Work out the finished part from the listing and answer in its coordinate system (mm). A direction names the side the tool comes from. Round coordinates to 2 decimals unless told otherwise and drop trailing zeros. Order: outer loops, then holes, each group sorted by start corner. A loop starts at its lowest first (then second) coordinate and runs counter-clockwise, first axis right, second up. Notation, with made-up numbers: (72.25, 29) - (80.25, 29) arc R32 ccw to (80.25, 62) - close; hole circle Ø9 at (62, 86.25). An arc over 180 degrees is marked (long way). Use CSV: the item, a comma, the result in double quotes.
from build123d import *

# Parameters (mm, degrees)
F1_DEPTH = 35
F2_W     = 220
F2_H     = 315
F3_DEPTH = 5


with BuildPart() as f1:
    # F0 (on Front) → F1 (new body)
    with BuildSketch(Plane.XZ):
        Polygon((-110, -157.5), (110, -157.5), (110, 157.5), (-110, 157.5), (-110, 152.500004), (105.000004, 152.500004), (105.000004, -152.500004), (-110, -152.500004), align=None)
    extrude(amount=F1_DEPTH)

    # F2 (on face) → F3 (join)
    with BuildSketch(Plane.XZ.offset(35)):
        Rectangle(F2_W, F2_H)
    extrude(amount=F3_DEPTH)


solid = f1.part
(1) Find the intervals of material crossed by L1, parallel to Z at x = -84.5, y = -26; L2, parallel to Y at x = -98, z = -5; L3, parallel to X at y = -19, z = -26, in increasing order. Write a range as from..to.
Findings below:
L1,"z = -157.5..-152.5, 152.5..157.5"
L2,"y = -40..-35"
L3,"x = 105..110"
(2) The mould has two halves that part along Z. Classify faces 3 (the flat face through (-2, -20, 157.5)), 4 (the flat face through (-4, -17, 152.5)), 5 (the flat face through (-2, -40, 2)): released by +Z, released by -Z, zero draft, split by the parting line, or undercut.
Findings below:
face 3,"released by +Z"
face 4,"undercut"
face 5,"zero draft"
(3) For faces 1 (the flat face through (105.4, 0, 0.7)), 2 (the flat face through (-1, -17, -152.5)), determine the directions among +Z, -Z, +X, -X, +Y, -Y from which every point of the face is accessible in a straight line to the end or side of a thin tool.
Findings below:
face 1,"+Z, -Z, +X, -X, +Y"
face 2,"-X, +Y"
(4) Find section C-C (z = -17.5). Determine the outline of the cut face in (x, y).
Findings below:
outline,"(-110, -40) - (110, -40) - (110, 0) - (105, 0) - (105, -35) - (-110, -35) - close"
(5) Find section B-B (y = -22). Determine the outline of the cut face in (x, z), and give its area (4 significant figures).
Findings below:
outline,"(-110, -157.5) - (110, -157.5) - (110, 157.5) - (-110, 157.5) - (-110, 152.5) - (105, 152.5) - (105, -152.5) - (-110, -152.5) - close"
area,"3,725 mm²"
(6) Each of these flat-tipped pins is pushed along its axis until it touches: pin 1 (12 mm diameter, centred on x = -74.5, z = 3.5, fed in from +Y); pin 2 (3 mm diameter, centred on y = -11, z = 41, fed in from -X). Where does it stop, or does it pass through?
Findings below:
pin 1,"stops at y = -35"
pin 2,"stops at x = 105"
(7) Find section A-A (x = 25.5). Determine the outline of the cut face in (y, z), and give its area (4 significant figures).
Findings below:
outline,"(-40, -157.5) - (0, -157.5) - (0, -152.5) - (-35, -152.5) - (-35, 152.5) - (0, 152.5) - (0, 157.5) - (-40, 157.5) - close"
area,"1,925 mm²"
